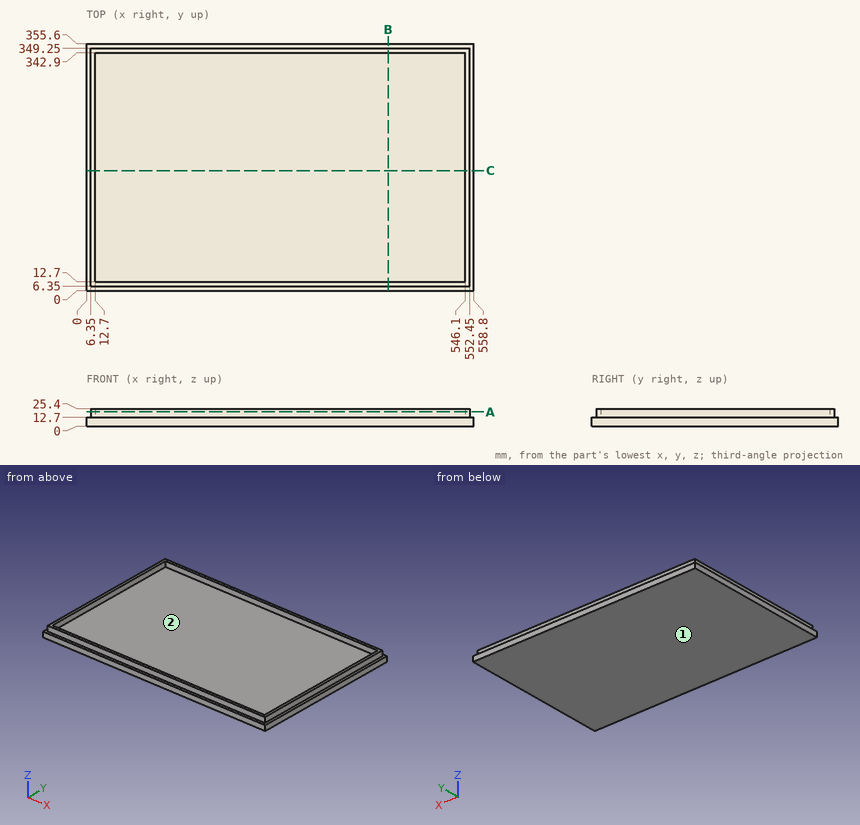
Source: three-view drawing plus pictorial views. Frame: mm from the lowest corner of the part. Round coordinates to 2 decimals unless told otherwise and drop trailing zeros. Write each loop counter-clockwise with the first axis right and the second up, starting at its lowest first coordinate (ties: lowest second). Pieces come first, ordered by that corner, then holes. Notation, with made-up numbers: M 85.5,80 L 144.5,80 A29 ccw 144.5,116 Z; hole C -38,-29 d7. An arc over 180 degrees is marked long. Write item = value, one per line.
Item 1: Pull-direction query (Y, two-part tool) for the marked faces 1 and 2; classes: pulls with the +Y half, pulls with the -Y half, needs draft (parallel to the pull), parting line crosses it, or undercut.
Findings:
face_1 = needs draft
face_2 = undercut
Item 2: Material intervals for line 1 along Y through (x, z) = (84, 20.5); line 2 along X through (y, z) = (23, 21); line 3 along Z through (x, y) = (228, 149.5), sorted ascending. Write a range as [from, to].
Findings:
line_1 = [6.35, 12.7], [342.9, 349.25]
line_2 = [6.35, 12.7], [546.1, 552.45]
line_3 = [0, 12.7]
Item 3: Pin query (flat end, axial travel): P1, Ø1, axis at x = 59, z = 4.5, coming from the -Y side; P2, Ø6.5, axis at x = 188.5, z = 20.5, coming from the -Y side; P3, Ø1.5, axis at y = 220, z = 13.5, coming from the +X side; P4, Ø4, axis at y = 223.5, z = 15, coming from the -X side. Return the tip coordinate at first contact, or that it passes through.
Findings:
P1 = 0
P2 = 6.35
P3 = 552.45
P4 = 6.35
Item 4: Section query C-C on y = 173. Return loops of the section in (x, z).
Findings:
outline = M 0,0 L 558.8,0 L 558.8,12.7 L 552.45,12.7 L 552.45,25.4 L 546.1,25.4 L 546.1,12.7 L 12.7,12.7 L 12.7,25.4 L 6.35,25.4 L 6.35,12.7 L 0,12.7 Z
Item 5: Section query B-B on x = 435. Return loops of the section in (y, z), then the cut area to 3 significant figures.
Findings:
outline = M 0,0 L 355.6,0 L 355.6,12.7 L 349.25,12.7 L 349.25,25.4 L 342.9,25.4 L 342.9,12.7 L 12.7,12.7 L 12.7,25.4 L 6.35,25.4 L 6.35,12.7 L 0,12.7 Z
area = 4,680 mm^2
Item 6: Section query A-A on z = 20.5. Return loops of the section in (x, y).
Findings:
outline = M 6.35,6.35 L 552.45,6.35 L 552.45,349.25 L 6.35,349.25 Z; hole M 12.7,12.7 L 546.1,12.7 L 546.1,342.9 L 12.7,342.9 Z
